```python
from build123d import *

# Parameters (mm, degrees)
SKETCH_1_R          = 29
EXTRUDE_1_DEPTH     = 122
CHAMFER_1_SIZE      = 3
SKETCH_2_R          = 4
EXTRUDE_2_DEPTH     = 30
CUT_EXTRUDE_START   = -15
CUT_EXTRUDE_1_DEPTH = 15


with BuildPart() as part:
    # Эскиз1 → Бобышка-Вытянуть1 (new body)
    with BuildSketch(Plane(origin=(0, 0, 0), x_dir=(0, 0, -1), z_dir=(1, 0, 0))):
        with Locations(Location((0, 0, 0), (0, 0, 180))):
            Circle(SKETCH_1_R)
    extrude(amount=EXTRUDE_1_DEPTH)

    # Фаска1
    chamfer_1_edges = [part.edges().sort_by_distance(p)[0] for p in [
        (0, 0, -29),
        (122, 0, -29),
    ]]
    chamfer(chamfer_1_edges, length=CHAMFER_1_SIZE)

    # Эскиз2 → Бобышка-Вытянуть2 (add)
    with BuildSketch(Plane(origin=(122, 0, 0), x_dir=(0, 0, -1), z_dir=(1, 0, 0))):
        Circle(SKETCH_2_R)
    extrude(amount=EXTRUDE_2_DEPTH)

    # Эскиз3 → Вырез-Вытянуть1 (cut)
    with BuildSketch(Plane(origin=(152, 0, 0), x_dir=(0, 0, -1), z_dir=(1, 0, 0)).offset(CUT_EXTRUDE_START)):
        with BuildLine():
            Line((-2.645751311, 3), (2.645751311, 3))
            ThreePointArc((2.645751311, 3), (0, 4), (-2.645751311, 3))
        make_face()
    extrude(amount=CUT_EXTRUDE_1_DEPTH, mode=Mode.SUBTRACT)


solid = part.part
```
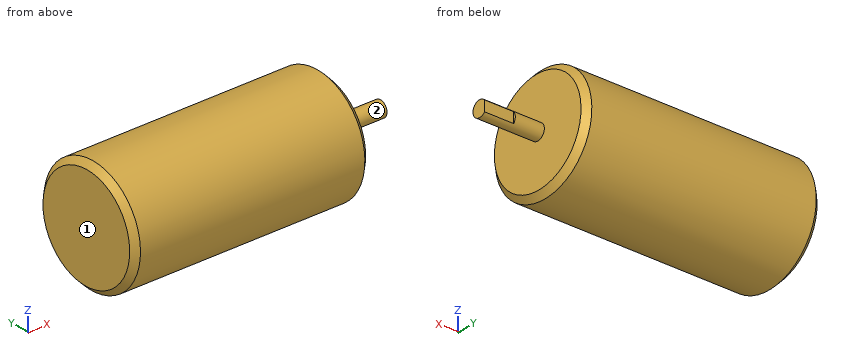
Check sheet for the modelled part. Datum: model origin and axes. Units: mm. Face numbers are marked on the shaded views. A direction names the side the tool comes from. Coordinates: 2 decimals unless noted, no trailing zeros. Loops run counter-clockwise (first coordinate to the right, second up) from the corner with the lowest first, then second, coordinate; pieces in that order, holes last.
1) Sectioned sample at A-A (y = 0). Record the boundary of the cut face in (x, z), and give its area (3 significant figures).
2) Sectioned sample at C-C (x = 131.5). Record the boundary of the cut face in (y, z).
3) Material ranges on probe 1 along X at (y, z) = (-21.5, -4); probe 2 along Y at (x, z) = (131, -3); probe 3 along Z at (x, y) = (52, -12.5), recorded low to high.
4) Access from +Z, -Z, +X, -X, +Y, -Y to the whole of each face (thin tool, end or side, straight path). Record for the marked faces 1 and 2.
5) Sectioned sample at B-B (z = 0). Record the boundary of the cut face in (x, y), and give its area (3 significant figures).
6) Sectioned sample at D-D (x = 59.5). Record the boundary of the cut face in (y, z).
7) Gauge pin test, flat ends, axial feed: pin 1 (3 mm diameter, centred on x = 47.5, z = -19, fed in from -Y); pin 2 (5 mm diameter, centred on x = 83.5, z = 10, fed in from -Y); pin 3 (4 mm diameter, centred on x = 146, z = 0.5, fed in from +Y). Record the tip position at first contact, or that the pin passes through.
Check sheet entries:
1. outline: (0, -26) - (3, -29) - (119, -29) - (122, -26) - (122, -4) - (152, -4) - (152, 4) - (122, 4) - (122, 26) - (119, 29) - (3, 29) - (0, 26) - close
1. area: 7,300 mm2
2. outline: circle Ø8 at (0, 0)
3. probe 1: x = 0 to 122
3. probe 2: y = -2.65 to 2.65
3. probe 3: z = -26.17 to 26.17
4. face 1: +Z, -Z, -X, +Y, -Y
4. face 2: +X
5. outline: (0, -26) - (3, -29) - (119, -29) - (122, -26) - (122, -4) - (152, -4) - (152, 3) - (137, 3) - (137, 4) - (122, 4) - (122, 26) - (119, 29) - (3, 29) - (0, 26) - close
5. area: 7,280 mm2
6. outline: circle Ø58 at (0, 0)
7. pin 1: stops at y = -23.12
7. pin 2: stops at y = -28.01
7. pin 3: stops at y = 3
